For this review, take the finished solid that the model builds, in its own axes (mm). A direction names the side the tool comes from. Coordinates: 2 decimals unless noted, no trailing zeros. Loops run counter-clockwise (first coordinate to the right, second up) from the corner with the lowest first, then second, coordinate; pieces in that order, holes last. Notation, with made-up numbers: (50, 76) - (69, 76) arc R19 ccw to (69, 106) - close; hole circle Ø7 at (62, 84.5). An arc over 180 degrees is marked (long way). One line per item, written item: value. Start each with the question number.
1. For faces 4 (the face through (254, 0, 13)), 5 (the face through (6, 14, 19.05)), list the 3-axis set-ups (+Z, -Z, +X, -X, +Y, -Y) from which the entire face can be reached by the end or side of a thin tool; tool diameter is ignored.
2. Take a section at D-D, the plane x = -156.5. State the section outline as (y, z) points, and give its area (3 significant figures).
3. Insertion check: pin 1 (7.5 mm diameter, centred on x = -2.5, y = 16.5, fed in from +Z); pin 2 (12.5 mm diameter, centred on x = 33, z = 17, fed in from +Y); pin 3 (14.5 mm diameter, centred on x = 228.6, z = 12.92, fed in from +Y). Each pin has a flat end and moves straight along its axis. Give the tip position at first contact, or say it passes through.
4. Take a section at B-B, the plane x = 0. State the section outline as (y, z) points, and give its area (3 significant figures).
5. To check wall thickness, follow line 1 (Z direction, x = 228.6, y = 1.25); line 2 (Y direction, x = -124.5, z = 8.25); line 3 (X direction, y = 0, z = 14.5). State the ranges of each line that lie inside material, in increasing order. Write a range as from..to.
6. Take a section at A-A, the plane x = -228.6. State the section outline as (y, z) points.
7. Take a section at C-C, the plane y = 16.51. State the section outline as (x, z) points.
8. The part is to be moulded in two halves that separate along Z. For faces 1 (the face through (0.526, 31.745, 22.181)), 2 (the face through (-234.944, -0.089, 13.201)), 3 (the face through (-4, 5, 25.4)), say which applies: released by +Z, released by -Z, zero draft, split by the parting line, or undercut.
```python
from build123d import *

# Parameters (mm, degrees)
F1_DEPTH = 25.4
F2_R     = 6.35
F3_DEPTH = 25.401
F4_W     = 41.7305262923
F4_H     = 12.7
F5_DEPTH = 508.001
F6_R     = 2.54
F7_R     = 6.35
F8_DEPTH = 38.101


with BuildPart() as f1:
    # F0 (on Top) → F1 (new body)
    with BuildSketch(Plane.XY):
        Polygon((-254, -6.35), (254, -6.35), (254, 6.35), (25.4, 6.35), (-25.4, 6.35), (-254, 6.35), align=None)
        with BuildLine():
            Line((-25.4, 6.35), (25.4, 6.35))
            ThreePointArc((25.4, 6.35), (0, 31.75), (-25.4, 6.35))
        make_face()
    extrude(amount=F1_DEPTH)

    # F2 (on face) → F3 (cut, through all)
    with BuildSketch(Plane.XY.offset(25.4)):
        with Locations((0, 16.51)):
            Circle(F2_R)
    extrude(amount=-F3_DEPTH, mode=Mode.SUBTRACT)

    # F4 (on face) → F5 (cut, through all)
    with BuildSketch(Plane(origin=(-254, 0, 0), x_dir=(0, -1, 0), z_dir=(-1, 0, 0))):
        with Locations((-27.2152631462, 12.7)):
            Rectangle(F4_W, F4_H)
    extrude(amount=-F5_DEPTH, mode=Mode.SUBTRACT)

    # F6
    f6_edges = [f1.edges().sort_by_distance(p)[0] for p in [
        (-25.4, 6.35, 3.175),
        (-25.4, 6.35, 22.225),
        (25.4, 6.35, 22.225),
        (25.4, 6.35, 3.175),
    ]]
    fillet(f6_edges, radius=F6_R)

    # F7 (on face) → F8 (cut, through all)
    with BuildSketch(Plane.XZ.offset(6.35)):
        with Locations((-228.6, 12.921767283)):
            Circle(F7_R)
        with Locations((228.6, 12.921767283)):
            Circle(F7_R)
    extrude(amount=-F8_DEPTH, mode=Mode.SUBTRACT)


solid = f1.part
```
Solutions:
1. face 4: +Z, -Z, +X, +Y, -Y
1. face 5: +X, -X, +Y
2. outline: (-6.35, 0) - (6.35, 0) - (6.35, 25.4) - (-6.35, 25.4) - close
2. area: 323 mm2
3. pin 1: through
3. pin 2: y = 6.46
3. pin 3: y = 6.35
4. outline: (-6.35, 0) - (10.16, 0) - (10.16, 6.35) - (6.35, 6.35) - (6.35, 19.05) - (10.16, 19.05) - (10.16, 25.4) - (-6.35, 25.4) - close; (22.86, 0) - (31.75, 0) - (31.75, 6.35) - (22.86, 6.35) - close; (22.86, 19.05) - (31.75, 19.05) - (31.75, 25.4) - (22.86, 25.4) - close
4. area: 484 mm2
5. line 1: 0..6.57, 19.27..25.4
5. line 2: -6.35..6.35
5. line 3: -254..-234.75, -222.45..222.45, 234.75..254
6. outline: (-6.35, 0) - (6.35, 0) - (6.35, 6.57) - (-6.35, 6.57) - close; (-6.35, 19.27) - (6.35, 19.27) - (6.35, 25.4) - (-6.35, 25.4) - close
7. outline: (-23.28, 0) - (-6.35, 0) - (-6.35, 6.35) - (-23.28, 6.35) - close; (-23.28, 19.05) - (-6.35, 19.05) - (-6.35, 25.4) - (-23.28, 25.4) - close; (6.35, 0) - (23.28, 0) - (23.28, 6.35) - (6.35, 6.35) - close; (6.35, 19.05) - (23.28, 19.05) - (23.28, 25.4) - (6.35, 25.4) - close
8. face 1: zero draft
8. face 2: undercut
8. face 3: released by +Z
